Verification items for the finished model (mm, model axes). A direction names the side the tool comes from. Give positions to 0.01 mm unless a question says otherwise; leave off trailing zeros. Loops run counter-clockwise (first coordinate to the right, second up) from the corner with the lowest first, then second, coordinate; pieces in that order, holes last. Notation, with made-up numbers: (7.5, 4.5) - (35.5, 4.5) arc R24 cw to (35.5, 29.5) - close; hole circle Ø10 at (51.25, 88). An arc over 180 degrees is marked (long way). One line per item, written item: value. Start each with the question number.
1. Sectioned sample at D-D (x = 2). Record the cut outline in (y, z).
2. Sectioned sample at C-C (x = -23). Record the cut outline in (y, z), plus the area to 3 significant figures.
3. Scan lines: L1, parallel to X at y = 10.4, z = 0; L2, parallel to Y at x = 11.5, z = -5.5; L3, parallel to Y at x = -25.5, z = 4.25. Record each from-to range of solid material in increasing order. Write a range as [from, to].
4. Sectioned sample at B-B (y = 10). Record the cut outline in (x, z).
5. Gauge pin test, flat ends, axial feed: pin 1 (5 mm diameter, centred on x = -0.5, z = 2, fed in from +Y); pin 2 (1 mm diameter, centred on y = -5, z = 5, fed in from +X); pin 3 (3.5 mm diameter, centred on x = 3, z = 0, fed in from -Y). Record the tip position at first contact, or that the pin passes through.
6. Sectioned sample at A-A (z = -3.5). Count the separate pieces of the cut face and the enclosed holes in it, plus the area to 3 significant figures.
7. Access from +Z, -Z, +X, -X, +Y, -Y to the whole of each face (thin tool, end or side, straight path). Record for faces 5 (the flat face through (1, 11.5, 0)), 6 (the flat face through (-21, 13, 5.5)), 7 (the flat face through (-27.001, 0, 0)).
8. Mould release check, pull along Y, two halves, no side actions. Record for faces 1 (the cylindrical face through (-11.286, -13.699, 0.112)), 2 (the flat face through (0, -9.5, 0)), 3 (the flat face through (-29.001, 0, 0)), 4 (the flat face through (-12.999, 11, 0)): pulls with the +Y half, pulls with the -Y half, needs draft (parallel to the pull), parting line crosses it, or undercut.
from build123d import *

# Parameters (mm, degrees)
Y_KSEKLIK_EKSTR_ZYON1_DEPTH = 8
IZIM2_R                     = 1.5
KES_EKSTR_ZYON1_DEPTH       = 18
IZIM3_W                     = 5
IZIM3_H                     = 2.5
KES_EKSTR_ZYON2_DEPTH       = 36


with BuildPart() as part:
    # Çizim1 → Yükseklik-Ekstrüzyon1 (new body, symmetric)
    with BuildSketch(Plane.XY):
        with BuildLine():
            ThreePointArc((-11.99936312, 14), (-11.292256338, 13.707106781), (-10.99936312, 13))
            Line((-10.99936312, 13), (-10.99936312, 12.499999979))
            ThreePointArc((-10.99936312, 12.499999979), (-10.706469901, 11.792893197), (-9.99936312, 11.499999979))
            Line((-9.99936312, 11.499999979), (13.00063688, 11.499999979))
            Line((13.00063688, 11.499999979), (13.00063688, 9.499999979))
            Line((13.00063688, 9.499999979), (-11.99936312, 9.499999979))
            ThreePointArc((-11.99936312, 9.499999979), (-12.706469901, 9.792893197), (-12.99936312, 10.499999979))
            Line((-12.99936312, 10.499999979), (-12.99936312, 12))
            Line((-12.99936312, 12), (-27.00063688, 12))
            Line((-27.00063688, 12), (-27.00063688, -12))
            Line((-27.00063688, -12), (-13.00063688, -12))
            Line((-13.00063688, -12), (-13.00063688, -10.499999979))
            ThreePointArc((-13.00063688, -10.499999979), (-12.707743662, -9.792893197), (-12.00063688, -9.499999979))
            Line((-12.00063688, -9.499999979), (12.99936312, -9.499999979))
            Line((12.99936312, -9.499999979), (12.99936312, -11.499999979))
            Line((12.99936312, -11.499999979), (-10.00063688, -11.499999979))
            ThreePointArc((-10.00063688, -11.499999979), (-10.707743662, -11.792893197), (-11.00063688, -12.499999979))
            Line((-11.00063688, -12.499999979), (-11.00063688, -13))
            ThreePointArc((-11.00063688, -13), (-11.293530099, -13.707106781), (-12.00063688, -14))
            Line((-12.00063688, -14), (-12.86760717, -14))
            Line((-12.86760717, -14), (-29.00063688, -14))
            Line((-29.00063688, -14), (-29.00063688, 14))
            Line((-29.00063688, 14), (-12.99936312, 14))
            Line((-12.99936312, 14), (-11.99936312, 14))
        make_face()
    extrude(amount=Y_KSEKLIK_EKSTR_ZYON1_DEPTH, both=True)

    # Çizim2 → Kes-Ekstrüzyon1 (cut, symmetric)
    with BuildSketch(Plane(origin=(0, 0, 0), x_dir=(1, 0, 0), z_dir=(0, 1, 0))):
        with Locations((3.00063688, 0)):
            Circle(IZIM2_R)
    extrude(amount=KES_EKSTR_ZYON1_DEPTH, both=True, mode=Mode.SUBTRACT)

    # Çizim3 → Kes-Ekstrüzyon2 (cut)
    with BuildSketch(Plane(origin=(0, 14, 0), x_dir=(1, 0, 0), z_dir=(0, 1, 0))):
        with Locations((-21.00063688, -4.25)):
            Rectangle(IZIM3_W, IZIM3_H)
        with Locations((-21.00063688, 4.25)):
            Rectangle(IZIM3_W, IZIM3_H)
    extrude(amount=-KES_EKSTR_ZYON2_DEPTH, mode=Mode.SUBTRACT)


solid = part.part
Results are:
1. outline: (-11.5, -8) - (-9.5, -8) - (-9.5, -1.12) - (-11.5, -1.12) - close; (-11.5, 1.12) - (-9.5, 1.12) - (-9.5, 8) - (-11.5, 8) - close; (9.5, -8) - (11.5, -8) - (11.5, -1.12) - (9.5, -1.12) - close; (9.5, 1.12) - (11.5, 1.12) - (11.5, 8) - (9.5, 8) - close
2. outline: (-14, -8) - (-12, -8) - (-12, -5.5) - (-14, -5.5) - close; (-14, -3) - (-12, -3) - (-12, 3) - (-14, 3) - close; (-14, 5.5) - (-12, 5.5) - (-12, 8) - (-14, 8) - close; (12, -8) - (14, -8) - (14, -5.5) - (12, -5.5) - close; (12, -3) - (14, -3) - (14, 3) - (12, 3) - close; (12, 5.5) - (14, 5.5) - (14, 8) - (12, 8) - close
2. area: 44.0 mm^2
3. L1: x = [-29, -27], [-12.99, 1.5], [4.5, 13]
3. L2: y = [-11.5, -9.5], [9.5, 11.5]
3. L3: y = [-14, -12], [12, 14]
4. outline: (-29, -8) - (-27, -8) - (-27, 8) - (-29, 8) - close; (-12.87, -8) - (13, -8) - (13, 8) - (-12.87, 8) - close; hole circle Ø3 at (3, 0)
5. pin 1: stops at y = 11.5
5. pin 2: stops at x = -27
5. pin 3: stops at y = -11.5
6. separate pieces: 3
6. enclosed holes: 0
6. area: 206 mm^2
7. face 5: +Z, -Z, +X, +Y
7. face 6: +Y, -Y
7. face 7: +Z, -Z
8. face 1: pulls with the -Y half
8. face 2: undercut
8. face 3: needs draft
8. face 4: undercut
